Source: CAD feature listing. Evaluate the final solid. Frame: model axes, mm. A direction names the side the tool comes from. Round coordinates to 2 decimals unless told otherwise and drop trailing zeros. Order: outer loops, then holes, each group sorted by start corner. A loop starts at its lowest first (then second) coordinate and runs counter-clockwise, first axis right, second up. Notation, with made-up numbers: (-15.5, 66.5) -> (13.5, 66.5) arc R21 cw to (13.5, 105.5) -> close; hole circle Ø2 at (43.5, 49). An arc over 180 degrees is marked (long way). Answer as CSV lines item,"result".
from build123d import *

# Parameters (mm, degrees)
BOSS_EXTRUDE1_DEPTH = 20
SKETCH2_R           = 1.75
BOSS_EXTRUDE2_DEPTH = 6
CUT_EXTRUDE1_DEPTH  = 20
BOSS_EXTRUDE3_DEPTH = 2
SKETCH5_W           = 10
SKETCH5_H           = 8.5
CUT_EXTRUDE2_DEPTH  = 3.5


with BuildPart() as part:
    # Sketch1 → Boss-Extrude1 (new body)
    with BuildSketch(Plane.XY):
        Polygon((0, 0), (0, 40), (-3, 40), (-10, 18), (-10, 0), align=None)
    extrude(amount=BOSS_EXTRUDE1_DEPTH)

    # Sketch2 → Boss-Extrude2 (add)
    with BuildSketch(Plane.XZ):
        Polygon((-10, 0), (-10, -10), (40, -10), (40, 0), (0, 0), align=None)
        with Locations(Location((35, -5, 0), (0, 0, 270))):
            Circle(SKETCH2_R, mode=Mode.SUBTRACT)
        with Locations(Location((5, -5, 0), (0, 0, 270))):
            Circle(SKETCH2_R, mode=Mode.SUBTRACT)
    extrude(amount=-BOSS_EXTRUDE2_DEPTH)

    # Sketch3 → Cut-Extrude1 (cut)
    with BuildSketch(Plane.XY.offset(20)):
        Polygon((0, 6), (-0.5, 6.5), (0, 7), align=None)
        Polygon((0, 7.5), (-0.5, 8), (0, 8.5), align=None)
        Polygon((0, 9), (-0.5, 9.5), (0, 10), align=None)
        Polygon((0, 10.5), (-0.5, 11), (0, 11.5), align=None)
        Polygon((0, 12), (-0.5, 12.5), (0, 13), align=None)
        Polygon((0, 13.5), (-0.5, 14), (0, 14.5), align=None)
        Polygon((0, 15), (-0.5, 15.5), (0, 16), align=None)
        Polygon((0, 16.5), (-0.5, 17), (0, 17.5), align=None)
        Polygon((0, 18), (-0.5, 18.5), (0, 19), align=None)
        Polygon((0, 19.5), (-0.5, 20), (0, 20.5), align=None)
        Polygon((0, 21), (-0.5, 21.5), (0, 22), align=None)
        Polygon((0, 22.5), (-0.5, 23), (0, 23.5), align=None)
        Polygon((0, 24), (-0.5, 24.5), (0, 25), align=None)
        Polygon((0, 25.5), (-0.5, 26), (0, 26.5), align=None)
        Polygon((0, 27), (-0.5, 27.5), (0, 28), align=None)
        Polygon((0, 28.5), (-0.5, 29), (0, 29.5), align=None)
        Polygon((0, 30), (-0.5, 30.5), (0, 31), align=None)
        Polygon((0, 31.5), (-0.5, 32), (0, 32.5), align=None)
        Polygon((0, 33), (-0.5, 33.5), (0, 34), align=None)
        Polygon((0, 34.5), (-0.5, 35), (0, 35.5), align=None)
        Polygon((0, 36), (-0.5, 36.5), (0, 37), align=None)
        Polygon((0, 37.5), (-0.5, 38), (0, 38.5), align=None)
        Polygon((0, 39), (-0.5, 39.5), (0, 40), align=None)
        Polygon((0, 40.5), (-0.5, 41), (0, 41.5), align=None)
    extrude(amount=-CUT_EXTRUDE1_DEPTH, mode=Mode.SUBTRACT)

    # Sketch4 → Boss-Extrude3 (add)
    # profile 1 of 2: a face of its own
    with BuildSketch(Plane(origin=(0, 6, 0), x_dir=(1, 0, 0), z_dir=(0, 1, 0))):
        Polygon((10.051814855, 5), (7.525907428, 9.375), (2.474092572, 9.375), (-0.051814855, 5), (2.474092572, 0.625), (7.525907428, 0.625), align=None)
        Polygon((9.474464586, 5), (7.237232293, 8.875), (2.762767707, 8.875), (0.525535414, 5), (2.762767707, 1.125), (7.237232293, 1.125), align=None, mode=Mode.SUBTRACT)
    # profile 2 of 2: a face of its own
    with BuildSketch(Plane(origin=(0, 6, 0), x_dir=(1, 0, 0), z_dir=(0, 1, 0))):
        Polygon((40.051814855, 5), (37.525907428, 9.375), (32.474092572, 9.375), (29.948185145, 5), (32.474092572, 0.625), (37.525907428, 0.625), align=None)
        Polygon((39.474464586, 5), (37.237232293, 8.875), (32.762767707, 8.875), (30.525535414, 5), (32.762767707, 1.125), (37.237232293, 1.125), align=None, mode=Mode.SUBTRACT)
    extrude(amount=BOSS_EXTRUDE3_DEPTH)

    # Sketch5 → Cut-Extrude2 (cut)
    with BuildSketch(Plane.XY.offset(20)):
        with Locations((-5, 4.25)):
            Rectangle(SKETCH5_W, SKETCH5_H)
    extrude(amount=-CUT_EXTRUDE2_DEPTH, mode=Mode.SUBTRACT)


solid = part.part
1. Mould query, pull axis X, two halves, no side actions, for faces 4 (the flat face through (9, 0, -2)), 5 (the flat face through (-10, 9, 9)), 6 (the flat face through (40, 3, -5)), 7 (the flat face through (38.37, 6.99, -6.91)). Classes: released by +X, released by -X, zero draft, split by the parting line, or undercut.
Results below:
face 4,"zero draft"
face 5,"released by -X"
face 6,"released by +X"
face 7,"undercut"
2. Section query B-B on x = 5. Return loops of the section in (y, z) (3 decimals), and give its area (3 significant figures).
Results below:
outline,"(0, -10) -> (6, -10) -> (6, -9.375) -> (8, -9.375) -> (8, -8.875) -> (6, -8.875) -> (6, -6.75) -> (0, -6.75) -> close; (0, -3.25) -> (6, -3.25) -> (6, -1.125) -> (8, -1.125) -> (8, -0.625) -> (6, -0.625) -> (6, 0) -> (0, 0) -> close"
area,"41.0 mm2"
3. Reachability of faces 1 (the flat face through (8.807, 6.986, -7.157)), 2 (the flat face through (5, 7, -9.375)), 3 (the flat face through (31.66, 6.986, -6.965)) from +Z, -Z, +X, -X, +Y, -Y: full face, straight path, thin tool, end or side. Return the list, or none.
Results below:
face 1,"-Z, +Y"
face 2,"-Z, +X, -X, +Y"
face 3,"+Y"
4. Section query C-C on x = -4. Return loops of the section in (y, z), and give its area (3 significant figures).
Results below:
outline,"(0, -10) -> (6, -10) -> (6, 0) -> (36.86, 0) -> (36.86, 20) -> (8.5, 20) -> (8.5, 16.5) -> (0, 16.5) -> close"
area,"767 mm2"
5. Section query A-A on y = 4. Return loops of the section in (x, z), and give its area (3 significant figures).
Results below:
outline,"(-10, -10) -> (40, -10) -> (40, 0) -> (0, 0) -> (0, 16.5) -> (-10, 16.5) -> close; hole circle Ø3.5 at (5, -5); hole circle Ø3.5 at (35, -5)"
area,"646 mm2"
6. Section query D-D on x = 20.5. Return loops of the section in (y, z).
Results below:
outline,"(0, -10) -> (6, -10) -> (6, 0) -> (0, 0) -> close"
7. Line query: L1, parallel to X at y = 2.65, z = -5; L2, parallel to Y at x = 26.5, z = -2.75; L3, parallel to X at y = 2, z = -8. Output: solid intervals per line, ascending. Write a range as [from, to].
Results below:
L1,"[-10, 3.25], [6.75, 33.25], [36.75, 40]"
L2,"[0, 6]"
L3,"[-10, 40]"
8. Pin query (flat end, axial travel): pin 1 (2.5 mm diameter, centred on x = -6, y = 6, fed in from +Z); pin 2 (0.6 mm diameter, centred on x = 35, y = 7, fed in from +Z) (3 decimals); pin 3 (4.5 mm diameter, centred on x = 37.5, z = -5.5, fed in from +Y); pin 4 (3 mm diameter, centred on x = 17.5, z = -4, fed in from -Y). Return the tip coordinate at first contact, or that it passes through.
Results below:
pin 1,"z = 16.5"
pin 2,"z = -0.625"
pin 3,"y = 8"
pin 4,"y = 0"
